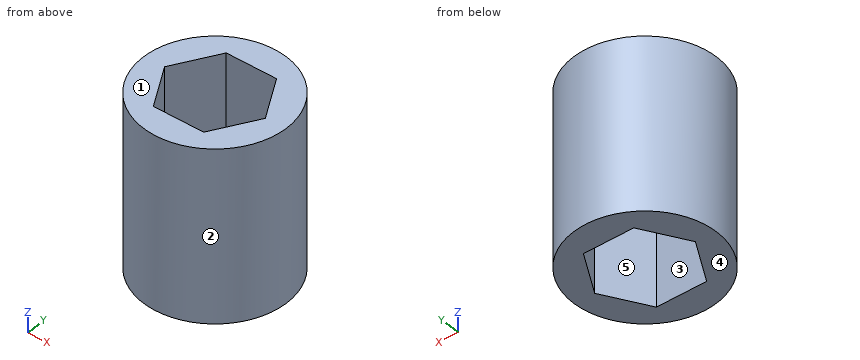
Autodesk Inventor part; units mm, degrees
ref_plane "YZ Plane" through (0, 0, 0) normal (1, 0, 0) x (0, 1, 0)
ref_plane "XZ Plane" through (0, 0, 0) normal (0, 1, 0) x (-1, 0, 0)
ref_plane "XY Plane" through (0, 0, 0) normal (0, 0, 1) x (1, 0, 0)
sketch "Sketch1" plane through (0, 0, 0) normal (0, 0, 1) x (1, 0, 0)
  line L0 (2.7496, 4.7625) -> (5.4993, 0)
  line L1 (5.4993, 0) -> (2.7496, -4.7625)
  line L2 (2.7496, -4.7625) -> (-2.7496, -4.7625)
  line L3 (-2.7496, -4.7625) -> (-5.4993, 0)
  line L4 (-5.4993, 0) -> (-2.7496, 4.7625)
  line L5 (-2.7496, 4.7625) -> (2.7496, 4.7625)
  circle A0 centre (0, 0) radius 7.9375
  circle A1 centre (0, 0) radius 5.4993 construction
  dimension "d0" = 9.525
  dimension "d2" = 15.875
  dimension "d3" = 2.4382
extrude "Extrusion1" add sketch "Sketch1" against normal blind 19.05
thicken "Thicken Hex" operation add thickness 0.127 both sides no extend neighbours yes toward (-0.8660254, 0.5, 0) faces at (-4.5827, 1.5875, -6.35) (-3.6662, -3.175, -6.35) (0.9165, -4.7625, -6.35) (-0.9165, 4.7625, -6.35) (3.6662, 3.175, -6.35) (4.5827, -1.5875, -6.35)
equation "\"d0\" = hexSize"
equation "\"d2\" = exteriorDiameter"
equation "\"d4\" = length"
equation "\"d6\" = printSpacing"
equation "\"d7\" = printSpacing"
equation "\"hexSize\" = 9.525"
equation "\"exteriorDiameter\" = 15.875"
equation "\"length\" = 19.05"
equation "\"printSpacing\" = 0.127"
properties part number "3_8x5_8x3_4-hexBearing" material "PC/ABS Plastic"
Can you work these out from the model? Positions are in its coordinate system, mm. Face numbers are marked on the shaded views. A direction names the side the tool comes from. Coordinates: 2 decimals unless noted, no trailing zeros. Write each loop counter-clockwise with the first axis right and the second up, starting at its lowest first coordinate (ties: lowest second). Pieces come first, ordered by that corner, then holes. Notation, with made-up numbers: M -7,27 L 1,27 A34 cw 1,64 Z; hole C 59.25,15.5 d4. An arc over 180 degrees is marked long. Write item = value, one per line. Start each with the question number.
Q1. I'm going to push flat-ended pins straight in: pin 1 (8 mm diameter, centred on x = 5.5, z = -17, fed in from -Y); pin 2 (8 mm diameter, centred on y = -5.5, z = -13, fed in from -X); pin 3 (1.5 mm diameter, centred on x = -1, z = -13.5, fed in from +Y). Where does each tip first touch, or does it pass through?
Q2. Thinking about a two-plate mould opening in Y: for the marked faces 1, 2 and 3, which applies, released by +Y, released by -Y, zero draft, split by the parting line, or undercut?
Q3. If we section it at C-C, the plane x = 0: Write out the boundary of the cut face in (y, z).
Q4. If we section it at B-B, the plane y = -2: Write out the boundary of the cut face in (x, z).
Q5. If I drill on L1, parallel to Y at x = 0.25, z = -15.5; L2, parallel to X at y = -1.75, z = -7; L3, parallel to X at y = 1, z = -15.5, over which ranges is the centre line in solid material (lowest first)? Write a range as [from, to].
Q6. If we section it at A-A, the plane z = -8.25: Write out the boundary of the cut face in (x, y) (1 decimal), then the cut area to 3 significant figures.
Q7. On a 3-axis mill with a long thin cutter (end or side, diameter ignored), from which of +Z, -Z, +X, -X, +Y, -Y can I reach the whole of each face in a straight line? I mean the marked faces 4 and 5. Say none if no direction works.
Check sheet entries:
q1.pin_1 = -7.79
q1.pin_2 = -7.79
q1.pin_3 = 7.93
q2.face_1 = zero draft
q2.face_2 = split by the parting line
q2.face_3 = undercut
q3.outline = M -7.94,-19.05 L -4.89,-19.05 L -4.89,0 L -7.94,0 Z; M 4.89,-19.05 L 7.94,-19.05 L 7.94,0 L 4.89,0 Z
q4.outline = M -7.68,-19.05 L -4.49,-19.05 L -4.49,0 L -7.68,0 Z; M 4.49,-19.05 L 7.68,-19.05 L 7.68,0 L 4.49,0 Z
q5.L1 = [-7.93, -4.89], [4.89, 7.93]
q5.L2 = [-7.74, -4.64], [4.64, 7.74]
q5.L3 = [-7.87, -5.07], [5.07, 7.87]
q6.outline = C 0,0 d15.9; hole M -5.6,0 L -2.8,-4.9 L 2.8,-4.9 L 5.6,0 L 2.8,4.9 L -2.8,4.9 Z
q6.area = 115 mm²
q7.face_4 = -Z, +X, -X, +Y, -Y
q7.face_5 = +Z, -Z
